```python
from build123d import *

# Parameters (mm, degrees)
F0_W     = 800
F0_H     = 400
F1_DEPTH = 200
F2_SIZE  = 50
F3_R     = 25
F4_R     = 25
F5_R     = 25
F7_D     = 100


with BuildPart() as f1:
    # F0 (on Front) → F1 (new body)
    with BuildSketch(Plane.XZ):
        Rectangle(F0_W, F0_H)
    extrude(amount=F1_DEPTH)

    # F2
    f2_edges = [f1.edges().sort_by_distance(p)[0] for p in [
        (-400, -200, 0),
        (-400, 0, 0),
    ]]
    chamfer(f2_edges, length=F2_SIZE)

    # F3
    f3_edges = [f1.edges().sort_by_distance(p)[0] for p in [
        (400, -100, -200),
    ]]
    fillet(f3_edges, radius=F3_R)

    # F4
    f4_edges = [f1.edges().sort_by_distance(p)[0] for p in [
        (400, -100, 200),
        (400, -200, 12.5),
    ]]
    fillet(f4_edges, radius=F4_R)

    # F5
    f5_edges = [f1.edges().sort_by_distance(p)[0] for p in [
        (400, 0, 0),
    ]]
    fillet(f5_edges, radius=F5_R)

    # F7 (through all)
    with Locations(Plane.XZ.offset(200)):
        with Locations((-86.828791, -3.877041)):
            Hole(F7_D / 2)


solid = f1.part
```
Geometry: final body of the model. Coordinates: model frame, mm. Round coordinates to 2 decimals unless told otherwise and drop trailing zeros. Write each loop counter-clockwise with the first axis right and the second up, starting at its lowest first coordinate (ties: lowest second). Pieces come first, ordered by that corner, then holes. Notation, with made-up numbers: (-23, 82.5) -> (13, 82.5) arc R28 ccw to (13, 108.5) -> close; hole circle Ø7 at (-14.5, 46.5). An arc over 180 degrees is marked (long way). Use CSV: the item, a comma, the result in double quotes. Start each with the question number.
Q1. Section A-A (z = -92). Return loops of the section in (x, y).
Q2. Section C-C (y = -14). Return loops of the section in (x, z), plus the area to 3 significant figures.
Q3. Line query: L1, parallel to Z at x = -107, y = -173; L2, parallel to X at y = -165, z = -11.5; L3, parallel to X at y = -126, z = 8.5. Output: solid intervals per line, ascending.
Q4. Section D-D (y = -134.5). Return loops of the section in (x, z), plus the area to 3 significant figures.
Q5. Section B-B (x = -110.5). Return loops of the section in (y, z), plus the area to 3 significant figures.
Q6. Pull-direction query (X, two-part tool) for faces 1 (the face through (392.871, -113.725, 192.482)), 2 (the face through (5.25, -7.129, -192.482)), 3 (the face through (-375, -175, -3)), 4 (the face through (-47.15, -98.6, -34.3)); classes: pulls with the +X half, pulls with the -X half, needs draft (parallel to the pull), parting line crosses it, or undercut.
Result sheet:
1,outline,"(-400, -150) -> (-350, -200) -> (375, -200) arc R25 ccw to (400, -175) -> (400, -25) arc R25 ccw to (375, 0) -> (-350, 0) -> (-400, -50) -> close"
2,outline,"(-364, -197.45) -> (375, -197.45) arc R22.45 ccw to (397.45, -175) -> (397.45, 175) arc R22.45 ccw to (375, 197.45) -> (-364, 197.45) -> close; hole circle Ø100 at (-86.83, -3.88)"
2,area,"293,000 mm²"
3,L1,"-200 to -49.63, 41.87 to 200"
3,L2,"-385 to -136.24, -37.41 to 400"
3,L3,"-400 to -135.27, -38.38 to 400"
4,outline,"(-400, -200) -> (375, -200) arc R25 ccw to (400, -175) -> (400, 175) arc R25 ccw to (375, 200) -> (-400, 200) -> close; hole circle Ø100 at (-86.83, -3.88)"
4,area,"312,000 mm²"
5,outline,"(-200, -175) arc R25 ccw to (-175, -200) -> (-25, -200) arc R25 ccw to (0, -175) -> (0, -47.92) -> (-200, -47.92) -> close; (-200, 40.16) -> (0, 40.16) -> (0, 175) arc R25 ccw to (-25, 200) -> (-200, 200) -> close"
5,area,"62,000 mm²"
6,face 1,"pulls with the +X half"
6,face 2,"needs draft"
6,face 3,"pulls with the -X half"
6,face 4,"undercut"
